Part model, mm, in its own coordinate system. Face numbers are marked on the shaded views. A direction names the side the tool comes from. Give positions to 0.01 mm unless a question says otherwise; leave off trailing zeros. Write each loop counter-clockwise with the first axis right and the second up, starting at its lowest first coordinate (ties: lowest second). Pieces come first, ordered by that corner, then holes. Notation, with made-up numbers: (7.25, 52.25) - (44.25, 52.25) arc R23 cw to (44.25, 82.25) - close; hole circle Ø1 at (-34, 57.5). An arc over 180 degrees is marked (long way). Answer as a JSON object with one key per item and string values. Group by question number.
```python
from build123d import *

# Parameters (mm, degrees)
F0_W     = 20
F0_H     = 15
F1_DEPTH = 15
F2_DEPTH = 25


with BuildPart() as f1:
    # F0 (on Top) → F1 (new body)
    with BuildSketch(Plane.XY):
        with Locations((10, -7.5)):
            Rectangle(F0_W, F0_H)
    extrude(amount=F1_DEPTH)

    # F0 (on Top) → F2 (join)
    with BuildSketch(Plane.XY):
        Polygon((20, -15), (0, -15), (-5, -22.5), (-5, -37.5), (2.5, -37.5), (2.5, -30), (17.5, -30), (17.5, -37.5), (25, -37.5), (25, -22.5), align=None)
    extrude(amount=F2_DEPTH)


solid = f1.part
```
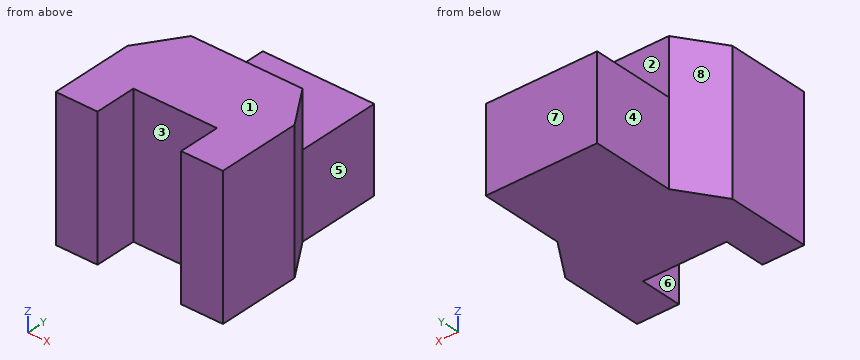
1) Band-saw the part on C-C (x = 19.5). List the corners of the cut face in (y, z).
2) Band-saw the part on B-B (z = 2.25). List the corners of the cut face in (x, y).
3) Probe line 1 (X direction, y = -36, z = 5.5); line 2 (X direction, y = -13.5, z = 4.5); line 3 (Y direction, x = 14.25, z = 8.75). List the from-to ranges inside material, lowest first.
4) Which spindle directions (+Z, -Z, +X, -X, +Y, -Y) get a long thin tool onto all of the face, cutting with end or side? Do the marked faces 1, 2, 3, 4 and 5. Say none if no direction does.
5) Drop flat-ended pins along their axis: P1, Ø7.5, axis at y = -8, z = 8.5, coming from the -X side; P2, Ø7.5, axis at y = -7.5, z = 6, coming from the +X side; P3, Ø7.5, axis at x = 9, y = -6.5, coming from the +Z side. Give the stop position or say it passes through.
6) Band-saw the part on A-A (y = -32). List the corners of the cut face in (x, z), plus the area to 3 significant figures.
7) Mould opens along X. For the marked faces 6, 7 and 8 say: pulls with the +X half, pulls with the -X half, needs draft (parallel to the pull), parting line crosses it, or undercut.
8) Band-saw the part on D-D (z = 15.75). List the corners of the cut face in (x, y), plus the area to 3 significant figures.
Verdict:
{
 "1": {"outline": "(-37.5, 0) - (0, 0) - (0, 15) - (-15, 15) - (-15, 25) - (-37.5, 25) - close"},
 "2": {"outline": "(-5, -37.5) - (2.5, -37.5) - (2.5, -30) - (17.5, -30) - (17.5, -37.5) - (25, -37.5) - (25, -22.5) - (20, -15) - (20, 0) - (0, 0) - (0, -15) - (-5, -22.5) - close"},
 "3": {"line 1": "-5 to 2.5, 17.5 to 25", "line 2": "0 to 20", "line 3": "-30 to 0"},
 "4": {"face 1": "+Z, +X, -X, +Y, -Y", "face 2": "+Z, +X, -X, +Y", "face 3": "+Z, -Z, -Y", "face 4": "+Z, -Z, -X, +Y", "face 5": "+Z, -Z, +X, +Y"},
 "5": {"P1": "x = 0", "P2": "x = 20", "P3": "z = 15"},
 "6": {"outline": "(-5, 0) - (2.5, 0) - (2.5, 25) - (-5, 25) - close; (17.5, 0) - (25, 0) - (25, 25) - (17.5, 25) - close", "area": "375 mm2"},
 "7": {"face 6": "undercut", "face 7": "needs draft", "face 8": "pulls with the -X half"},
 "8": {"outline": "(-5, -37.5) - (2.5, -37.5) - (2.5, -30) - (17.5, -30) - (17.5, -37.5) - (25, -37.5) - (25, -22.5) - (20, -15) - (0, -15) - (-5, -22.5) - close", "area": "525 mm2"}
}
